Read the model definition and answer for the solid it produces. Units are mm, in the model's axes. Face numbers are marked on the shaded views. A direction names the side the tool comes from. Coordinates: 2 decimals unless noted, no trailing zeros. Write each loop counter-clockwise with the first axis right and the second up, starting at its lowest first coordinate (ties: lowest second). Pieces come first, ordered by that corner, then holes.
(1) Which of the six approach directions +Z, -Z, +X, -X, +Y, -Y give full straight-line access (tool end or side, diameter ignored) to the marked faces 4, 5, 6, 7 and 8?
(2) The part is cut by section D-D, the plane x = 11. Determine the outline of the cut face in (y, z), and give its area (3 significant figures).
(3) Determine the mould class of the marked faces 1, 2 and 3 for opening direction X: pulls with the +X half, pulls with the -X half, needs draft (parallel to the pull), parting line crosses it, or undercut.
(4) The part is cut by section A-A, the plane x = -2.5. Determine the outline of the cut face in (y, z), and give its area (3 significant figures).
(5) The part is cut by section C-C, the plane y = 2.25. Determine the outline of the cut face in (x, z).
(6) Straight lines are drawn through the part: line 1 along Z through (x, y) = (2, 1); line 2 along X through (y, z) = (1, -6); line 3 along Y through (x, z) = (-6.5, 8). For each, find the intervals that lie inside material, in ascending order.
(7) Given pin 1 (3 mm diameter, centred on y = 6.5, z = 3.5, fed in from +X); pin 2 (0.6 mm diameter, centred on x = -12.5, z = 1.5, fed in from +Y); pin 3 (2 mm diameter, centred on y = 9.5, z = 0, fed in from -X); pin 4 (6 mm diameter, centred on x = -6.5, z = -1, fed in from +Y), each flat-ended and moving along its own axis, determine where each tip first touches the part or whether it passes through.
(8) The part is cut by section B-B, the plane z = 3. Determine the outline of the cut face in (x, y), and give its area (3 significant figures).
```python
from build123d import *

# Parameters (mm, degrees)
SKETCH1_W           = 40
SKETCH1_H           = 20
BOSS_EXTRUDE1_DEPTH = 4
SKETCH2_W           = 16.25
SKETCH2_H           = 14.5
CUT_EXTRUDE2_DEPTH  = 3.5
SKETCH3_W           = 15.25
SKETCH3_H           = 14.5
CUT_EXTRUDE3_DEPTH  = 0.5
SKETCH4_W           = 2
SKETCH4_H           = 14.5
BOSS_EXTRUDE2_DEPTH = 6
FILLET1_R           = 4
FILLET2_R           = 0.5
SKETCH5_W           = 2.5
SKETCH5_H           = 14.5
BOSS_EXTRUDE3_DEPTH = 4.4
SKETCH6_W           = 4.6
SKETCH6_H           = 14.5
BOSS_EXTRUDE4_DEPTH = 2.5
BOSS_EXTRUDE5_DEPTH = 14.5
FILLET3_R           = 1
FILLET4_R           = 4


with BuildPart() as part:
    # Sketch1 → Boss-Extrude1 (new body)
    with BuildSketch(Plane(origin=(0, 0, 0), x_dir=(1, 0, 0), z_dir=(0, 1, 0))):
        Rectangle(SKETCH1_W, SKETCH1_H)
    extrude(amount=BOSS_EXTRUDE1_DEPTH)

    # Sketch2 → Cut-Extrude2 (cut)
    with BuildSketch(Plane(origin=(0, 4, 0), x_dir=(1, 0, 0), z_dir=(0, 1, 0))):
        with Locations((-2.875, 0)):
            Rectangle(SKETCH2_W, SKETCH2_H)
    extrude(amount=-CUT_EXTRUDE2_DEPTH, mode=Mode.SUBTRACT)

    # Sketch3 → Cut-Extrude3 (cut)
    with BuildSketch(Plane(origin=(0, 0.5, 0), x_dir=(1, 0, 0), z_dir=(0, 1, 0))):
        with Locations((-3.375, 0)):
            Rectangle(SKETCH3_W, SKETCH3_H)
    extrude(amount=-CUT_EXTRUDE3_DEPTH, mode=Mode.SUBTRACT)

    # Sketch4 → Boss-Extrude2 (add)
    with BuildSketch(Plane(origin=(0, 4, 0), x_dir=(1, 0, 0), z_dir=(0, 1, 0))):
        with Locations((-13.15, 0)):
            Rectangle(SKETCH4_W, SKETCH4_H)
    extrude(amount=BOSS_EXTRUDE2_DEPTH)

    # Fillet1
    fillet1_edges = [part.edges().sort_by_distance(p)[0] for p in [
        (-14.15, 4, 0),
    ]]
    fillet(fillet1_edges, radius=FILLET1_R)

    # Fillet2
    fillet2_edges = [part.edges().sort_by_distance(p)[0] for p in [
        (-12.15, 4, 0),
    ]]
    fillet(fillet2_edges, radius=FILLET2_R)

    # Sketch5 → Boss-Extrude3 (add)
    with BuildSketch(Plane(origin=(0, 4, 0), x_dir=(1, 0, 0), z_dir=(0, 1, 0))):
        with Locations((11.5, 0)):
            Rectangle(SKETCH5_W, SKETCH5_H)
    extrude(amount=BOSS_EXTRUDE3_DEPTH)

    # Sketch6 → Boss-Extrude4 (add)
    with BuildSketch(Plane(origin=(0, 8.4, 0), x_dir=(1, 0, 0), z_dir=(0, 1, 0))):
        with Locations((10.45, 0)):
            Rectangle(SKETCH6_W, SKETCH6_H)
    extrude(amount=BOSS_EXTRUDE4_DEPTH)

    # Sketch7 → Boss-Extrude5 (add)
    with BuildSketch(Plane.XY.offset(7.25)):
        Polygon((12.75, 4), (15.25, 4), (12.75, 10.9), align=None)
    extrude(amount=-BOSS_EXTRUDE5_DEPTH)

    # Fillet3
    fillet3_edges = [part.edges().sort_by_distance(p)[0] for p in [
        (12.75, 10.9, 0),
    ]]
    fillet(fillet3_edges, radius=FILLET3_R)

    # Fillet4
    fillet4_edges = [part.edges().sort_by_distance(p)[0] for p in [
        (15.25, 4, 0),
    ]]
    fillet(fillet4_edges, radius=FILLET4_R)


solid = part.part
```
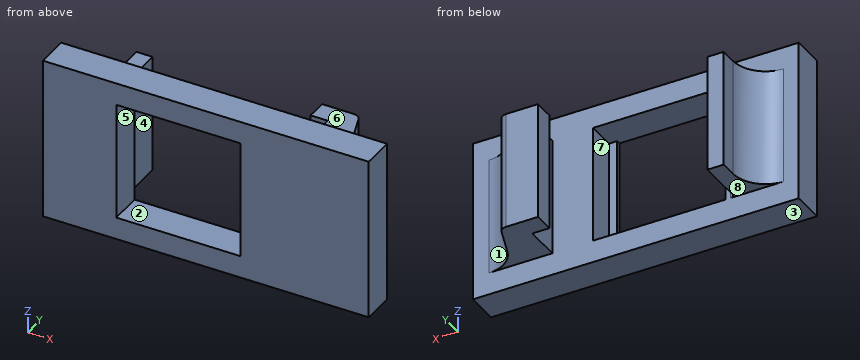
Computed:
1. face 4: +Z, -Z, +Y
1. face 5: +Y, -Y
1. face 6: +Z, +X, -X, +Y
1. face 7: +Y
1. face 8: -Z, +X, -X, +Y
2. outline: (0, -10) - (4, -10) - (4, -7.25) - (10.9, -7.25) - (10.9, 7.25) - (4, 7.25) - (4, 10) - (0, 10) - close
2. area: 180 mm2
3. face 1: pulls with the +X half
3. face 2: undercut
3. face 3: needs draft
4. outline: (0, -10) - (4, -10) - (4, -7.25) - (0, -7.25) - close; (0, 7.25) - (4, 7.25) - (4, 10) - (0, 10) - close
4. area: 22.0 mm2
5. outline: (-20, -10) - (20, -10) - (20, 10) - (-20, 10) - close; hole (-11, -7.25) - (5.25, -7.25) - (5.25, 7.25) - (-11, 7.25) - close
6. line 1: z = -10 to -7.25, 7.25 to 10
6. line 2: x = -20 to -11, 5.25 to 20
6. line 3: y = 0 to 4
7. pin 1: stops at x = 15.41
7. pin 2: stops at y = 10
7. pin 3: stops at x = -14.15
7. pin 4: passes through
8. outline: (-20, 0) - (-11, 0) - (-11, 4) - (-11.65, 4) arc R0.5 cw to (-12.15, 4.5) - (-12.15, 10) - (-14.15, 10) - (-14.15, 8) arc R4 cw to (-18.15, 4) - (-20, 4) - close; (4.25, 0) - (20, 0) - (20, 4) - (18.06, 4) arc R4 cw to (14.29, 6.64) - (12.99, 10.24) arc R1 ccw to (12.05, 10.9) - (8.15, 10.9) - (8.15, 8.4) - (10.25, 8.4) - (10.25, 4) - (5.25, 4) - (5.25, 0.5) - (4.25, 0.5) - close
8. area: 143 mm2
